Here's how the part is built. I have some questions about the finished solid (model axes, mm). Round coordinates to 2 decimals unless told otherwise and drop trailing zeros. Loops run counter-clockwise (first coordinate to the right, second up) from the corner with the lowest first, then second, coordinate; pieces in that order, holes last. Notation, with made-up numbers: (-14, 25.25) -> (0, 25.25) arc R27 cw to (0, 59.25) -> close; hole circle Ø6 at (20, 31). An arc over 180 degrees is marked (long way). One line per item, written item: value. Start each with the question number.
```python
from build123d import *

# Parameters (mm, degrees)
SKETCH1_W           = 45
SKETCH1_H           = 30
SKETCH1_R           = 7.5
BOSS_EXTRUDE1_DEPTH = 25
CHAMFER1_SIZE       = 1


with BuildPart() as part:
    # Sketch1 → Boss-Extrude1 (new body, symmetric)
    with BuildSketch(Plane.XY):
        Rectangle(SKETCH1_W, SKETCH1_H)
        with Locations((-10, 0)):
            Circle(SKETCH1_R, mode=Mode.SUBTRACT)
        with Locations((10, 0)):
            Circle(SKETCH1_R, mode=Mode.SUBTRACT)
    extrude(amount=BOSS_EXTRUDE1_DEPTH, both=True)

    # Chamfer1
    chamfer1_edges = [part.edges().sort_by_distance(p)[0] for p in [
        (-17.5, 0, -25),
        (-17.5, 0, 25),
        (2.5, 0, -25),
        (2.5, 0, 25),
    ]]
    chamfer(chamfer1_edges, length=CHAMFER1_SIZE)


solid = part.part
```
Q1. I want a section at A-A on y = 0. Please give me the cut outline in (x, z), plus the area to 3 significant figures.
Q2. I want a section at B-B on x = 10. Please give me the cut outline in (y, z), plus the area to 3 significant figures.
Q3. I want a section at D-D on y = -4.25. State how many separate pieces and enclosed holes the cut face has, plus the area to 3 significant figures.
Q4. If we mould it in two halves opening along Y, with no side actions, what happens to faces 1 (the flat face through (0, -15, 0)), 2 (the flat face through (22.5, 0, 0)), 3 (the cylindrical face through (2.507, 0.33, -0.336))? For each: released by +Y, released by -Y, zero draft, split by the parting line, or undercut.
Q5. I want a section at C-C on z = -21. Please give me the cut outline in (x, y), plus the area to 3 significant figures.
Q6. Will this pin go through, and if not, where does the flat tip stop? P1, Ø3, axis at x = -9.5, y = 6.5, coming from the +Z side.
Q7. If I drill on line 1 along Y through (x, z) = (10, 14); line 2 along X through (y, z) = (-5.25, -16.5); line 3 along X through (y, z) = (3.75, 7.5), over which ranges is the centre line in solid material (lowest first)?
Answers below:
1. outline: (-22.5, -25) -> (-18.5, -25) -> (-17.5, -24) -> (-17.5, 24) -> (-18.5, 25) -> (-22.5, 25) -> close; (-2.5, -24) -> (-1.5, -25) -> (1.5, -25) -> (2.5, -24) -> (2.5, 24) -> (1.5, 25) -> (-1.5, 25) -> (-2.5, 24) -> close; (17.5, -24) -> (18.5, -25) -> (22.5, -25) -> (22.5, 25) -> (18.5, 25) -> (17.5, 24) -> close
1. area: 746 mm^2
2. outline: (-15, -25) -> (-8.5, -25) -> (-7.5, -24) -> (-7.5, 24) -> (-8.5, 25) -> (-15, 25) -> close; (7.5, -24) -> (8.5, -25) -> (15, -25) -> (15, 25) -> (8.5, 25) -> (7.5, 24) -> close
2. area: 748 mm^2
3. separate pieces: 3
3. enclosed holes: 0
3. area: 1,010 mm^2
4. face 1: released by -Y
4. face 2: zero draft
4. face 3: undercut
5. outline: (-22.5, -15) -> (22.5, -15) -> (22.5, 15) -> (-22.5, 15) -> close; hole circle Ø15 at (-10, 0); hole circle Ø15 at (10, 0)
5. area: 997 mm^2
6. P1: stops at z = 24.52
7. line 1: y = -15 to -7.5, 7.5 to 15
7. line 2: x = -22.5 to -15.36, -4.64 to 4.64, 15.36 to 22.5
7. line 3: x = -22.5 to -16.5, -3.5 to 3.5, 16.5 to 22.5
